Check sheet for the modelled part. Datum: model origin and axes. Units: mm. Face numbers are marked on the shaded views. A direction names the side the tool comes from. Give positions to 0.01 mm unless a question says otherwise; leave off trailing zeros. Order: outer loops, then holes, each group sorted by start corner. A loop starts at its lowest first (then second) coordinate and runs counter-clockwise, first axis right, second up.
```python
from build123d import *

# Parameters (mm, degrees)
CROQUIS1_R              = 1.75
SALIENTE_EXTRUIR1_DEPTH = 4
CROQUIS2_W              = 30.8
CROQUIS2_H              = 4.2
SALIENTE_EXTRUIR2_DEPTH = 4
CROQUIS3_W              = 8.5
CROQUIS3_H              = 20.5
CORTAR_EXTRUIR1_DEPTH   = 4
REDONDEO1_R             = 4
REDONDEO2_R             = 4
CHAFL_N1_SIZE           = 1
CROQUIS4_R              = 2.9
CORTAR_EXTRUIR2_DEPTH   = 1
REDONDEO3_R             = 5


with BuildPart() as part:
    # Croquis1 → Saliente-Extruir1 (new body)
    with BuildSketch(Plane(origin=(0, 0, 0), x_dir=(1, 0, 0), z_dir=(0, 1, 0))):
        Polygon((0, 0), (0, 45), (45, 45), (45, 35), (10, 35), (10, 0), align=None)
        with Locations(Location((35, 40, 0), (0, 0, 270))):
            Circle(CROQUIS1_R, mode=Mode.SUBTRACT)
        with Locations(Location((5, 10, 0), (0, 0, 270))):
            Circle(CROQUIS1_R, mode=Mode.SUBTRACT)
    extrude(amount=SALIENTE_EXTRUIR1_DEPTH)

    # Croquis2 → Saliente-Extruir2 (add)
    with BuildSketch(Plane(origin=(0, 4, 0), x_dir=(1, 0, 0), z_dir=(0, 1, 0))):
        with Locations((29.6, 32.9)):
            Rectangle(CROQUIS2_W, CROQUIS2_H)
        Polygon((10, 35), (10, 0), (14.2, 0), (14.2, 30.8), (14.2, 35), align=None)
    extrude(amount=-SALIENTE_EXTRUIR2_DEPTH)

    # Croquis3 → Cortar-Extruir1 (cut)
    with BuildSketch(Plane(origin=(0, 4, 0), x_dir=(1, 0, 0), z_dir=(0, 1, 0))):
        Polygon((29, 45), (0, 45), (0, 36.5), (8.5, 36.5), (29, 36.5), align=None)
        with Locations((4.25, 26.25)):
            Rectangle(CROQUIS3_W, CROQUIS3_H)
    extrude(amount=-CORTAR_EXTRUIR1_DEPTH, mode=Mode.SUBTRACT)

    # Redondeo1
    redondeo1_edges = [part.edges().sort_by_distance(p)[0] for p in [
        (14.2, 2, -30.8),
        (8.5, 2, -36.5),
    ]]
    fillet(redondeo1_edges, radius=REDONDEO1_R)

    # Redondeo2
    redondeo2_edges = [part.edges().sort_by_distance(p)[0] for p in [
        (0, 2, 0),
        (45, 2, -45),
        (0, 2, -16),
        (29, 2, -45),
    ]]
    fillet(redondeo2_edges, radius=REDONDEO2_R)

    # Chaflán1
    chafl_n1_edges = [part.edges().sort_by_distance(p)[0] for p in [
        (31.6, 4, -30.8),
        (14.2, 4, -13.4),
        (15.371572875, 4, -29.628427125),
    ]]
    chamfer(chafl_n1_edges, length=CHAFL_N1_SIZE)

    # Croquis4 → Cortar-Extruir2 (cut)
    with BuildSketch(Plane(origin=(0, 4, 0), x_dir=(1, 0, 0), z_dir=(0, 1, 0))):
        with Locations(Location((35, 40, 0), (0, 0, 270))):
            Circle(CROQUIS4_R)
        with Locations(Location((5, 10, 0), (0, 0, 270))):
            Circle(CROQUIS4_R)
    extrude(amount=-CORTAR_EXTRUIR2_DEPTH, mode=Mode.SUBTRACT)

    # Redondeo3
    redondeo3_edges = [part.edges().sort_by_distance(p)[0] for p in [
        (8.5, 2, -16),
        (29, 2, -36.5),
    ]]
    fillet(redondeo3_edges, radius=REDONDEO3_R)


solid = part.part
```
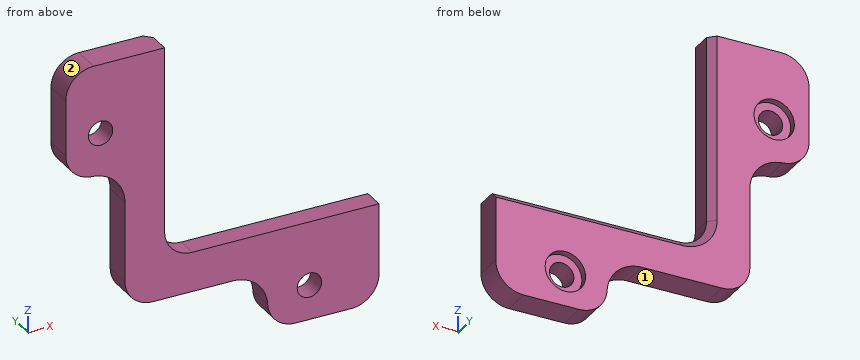
Q1. Tool access check on the marked faces 1 and 2. Record the directions out of +Z, -Z, +X, -X, +Y, -Y that give a thin tool (end or side, any length) a straight path to the whole face; none if there is none.
Q2. Sectioned sample at D-D, the plane z = -26. Record the cut outline in (x, y), plus the area to 3 significant figures.
Q3. Sectioned sample at C-C, the plane y = 1.75. Count the separate pieces of the cut face and the enclosed holes in it, plus the area to 3 significant figures.
Q4. Sectioned sample at A-A, the plane z = -10. Record the cut outline in (x, y), plus the area to 3 significant figures.
Q5. Sectioned sample at B-B, the plane x = 20.5. Record the cut outline in (y, z), plus the area to 3 significant figures.
Q6. Material ranges on line 1 (Z direction, x = 35, y = 2.3); line 2 (Z direction, x = 22.5, y = 2.2); line 3 (X direction, y = 2, z = -31), recorded low to high.
Q7. Go/stop test with flat-tipped pins: P1, Ø1.2, axis at y = 2.5, z = -25, coming from the -X side; P2, Ø3, axis at x = 35, z = -40, coming from the -Y side; P3, Ø4.5, axis at x = 5, z = -10, coming from the +Y side; P4, Ø0.9, axis at y = 2, z = -18, coming from the +X side. Record where each tip stops, or that it passes through.
Filled in:
1. face 1: -Z, -X, +Y, -Y
1. face 2: +Z, -X, +Y, -Y
2. outline: (8.5, 0) - (14.2, 0) - (14.2, 3) - (13.2, 4) - (8.5, 4) - close
2. area: 22.3 mm2
3. separate pieces: 1
3. enclosed holes: 2
3. area: 633 mm2
4. outline: (0, 0) - (3.25, 0) - (3.25, 3) - (2.1, 3) - (2.1, 4) - (0, 4) - close; (6.75, 0) - (14.2, 0) - (14.2, 3) - (13.2, 4) - (7.9, 4) - (7.9, 3) - (6.75, 3) - close
4. area: 40.0 mm2
5. outline: (0, -36.5) - (4, -36.5) - (4, -31.8) - (3, -30.8) - (0, -30.8) - close
5. area: 22.3 mm2
6. line 1: z = -45 to -41.75, -38.25 to -30.8
6. line 2: z = -36.5 to -30.8
6. line 3: x = 8.5 to 45
7. P1: stops at x = 8.5
7. P2: passes through
7. P3: stops at y = 3
7. P4: stops at x = 14.2
